```python
from build123d import *

# Parameters (mm, degrees)
ESQUISSE1_W        = 8
ESQUISSE1_H        = 8
ESQUISSE1_R        = 2.825
BOSS_EXTRU_1_DEPTH = 6


with BuildPart() as part:
    # Esquisse1 → Boss.-Extru.1 (new body)
    # profile 1 of 6: a face of its own
    with BuildSketch(Plane(origin=(0, 0, 0), x_dir=(1, 0, 0), z_dir=(0, 1, 0))):
        Rectangle(ESQUISSE1_W, ESQUISSE1_H)
        Circle(ESQUISSE1_R, mode=Mode.SUBTRACT)
    # profile 2 of 6: a face of its own
    with BuildSketch(Plane(origin=(0, 0, 0), x_dir=(1, 0, 0), z_dir=(0, 1, 0))):
        Polygon((1.6, -4), (-1.6, -4), (0, -5.7), align=None)
    # profile 3 of 6: a face of its own
    with BuildSketch(Plane(origin=(0, 0, 0), x_dir=(1, 0, 0), z_dir=(0, 1, 0))):
        Polygon((-1.6, 4), (-4, 4), (-4, 1.6), (-4, -1.6), (-4, -4), (-1.6, -4), (1.6, -4), (4, -4), (4, 4), (1.6, 4), align=None)
        with BuildLine():
            ThreePointArc((1.708252031, -2.25), (-2.825, 0), (1.708252031, 2.25))
            ThreePointArc((1.708252031, 2.25), (2.530458159, 1.255948449), (2.825, 0))
            ThreePointArc((2.825, 0), (2.530458159, -1.255948449), (1.708252031, -2.25))
        make_face(mode=Mode.SUBTRACT)
    # profile 4 of 6: a face of its own
    with BuildSketch(Plane(origin=(0, 0, 0), x_dir=(1, 0, 0), z_dir=(0, 1, 0))):
        with BuildLine():
            ThreePointArc((2.825, 0), (2.530458159, 1.255948449), (1.708252031, 2.25))
            Line((1.708252031, 2.25), (1.708252031, -2.25))
            ThreePointArc((1.708252031, -2.25), (2.530458159, -1.255948449), (2.825, 0))
        make_face()
    # profile 5 of 6: a face of its own
    with BuildSketch(Plane(origin=(0, 0, 0), x_dir=(1, 0, 0), z_dir=(0, 1, 0))):
        Polygon((-4, -1.6), (-4, 1.6), (-5.7, 0), align=None)
    # profile 6 of 6: a face of its own
    with BuildSketch(Plane(origin=(0, 0, 0), x_dir=(1, 0, 0), z_dir=(0, 1, 0))):
        Polygon((0, 5.7), (-1.6, 4), (1.6, 4), align=None)
    extrude(amount=BOSS_EXTRU_1_DEPTH)


solid = part.part
```
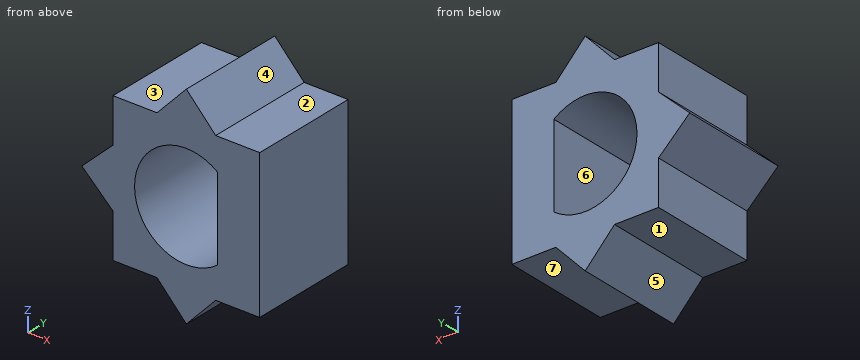
Could you check a few things on this model? Use its own coordinates, in mm. Face numbers are marked on the shaded views. A direction names the side the tool comes from. Round coordinates to 2 decimals unless told otherwise and drop trailing zeros. Loops run counter-clockwise (first coordinate to the right, second up) from the corner with the lowest first, then second, coordinate; pieces in that order, holes last. Notation, with made-up numbers: (7.25, 75.25) - (18.25, 75.25) arc R27 ccw to (18.25, 100.25) - close; hole circle Ø3 at (56.25, 68.25). An arc over 180 degrees is marked (long way). Use CSV: the item, a comma, the result in double quotes.
Item 1: If we section it at C-C on y = 1.5: List the corners of the cut face in (x, z) for me (3 decimals), then the cut area to 3 significant figures.
Here are the results:
outline,"(-5.7, 0) - (-4, -1.6) - (-4, -4) - (-1.6, -4) - (0, -5.7) - (1.6, -4) - (4, -4) - (4, 4) - (1.6, 4) - (0, 5.7) - (-1.6, 4) - (-4, 4) - (-4, 1.6) - close; hole (1.708, -2.25) - (1.708, 2.25) arc R2.825 ccw (long way) to start"
area,"50.6 mm²"
Item 2: If we section it at D-D on z = 4.75: List the corners of the cut face in (x, y) for me, then the cut area to 3 significant figures.
Here are the results:
outline,"(-0.89, 0) - (0.89, 0) - (0.89, 6) - (-0.89, 6) - close"
area,"10.7 mm²"
Item 3: If we section it at A-A on x = -0.75: List the corners of the cut face in (y, z) for me, then the cut area to 3 significant figures.
Here are the results:
outline,"(0, -4.9) - (6, -4.9) - (6, -2.72) - (0, -2.72) - close; (0, 2.72) - (6, 2.72) - (6, 4.9) - (0, 4.9) - close"
area,"26.2 mm²"
Item 4: For the marked faces 1, 2 and 3, which set-ups out of +Z, -Z, +X, -X, +Y, -Y let a thin tool reach every point of the face, with its end or its side?
Here are the results:
face 1,"-Z, -X, +Y, -Y"
face 2,"+Z, +X, +Y, -Y"
face 3,"+Z, -X, +Y, -Y"
Item 5: I need wall thicknesses on L1, parallel to Z at x = 3.5, y = 5.7; L2, parallel to Z at x = 0.25, y = 2.1; L3, parallel to Z at x = -2, y = 3. Which ranges of each line are inside material? Lowest first, please. Write a range as [from, to].
Here are the results:
L1,"z = [-4, 4]"
L2,"z = [-5.43, -2.81], [2.81, 5.43]"
L3,"z = [-4, -2], [2, 4]"
Item 6: If we section it at B-B on z = -1.25: List the corners of the cut face in (x, y) for me.
Here are the results:
outline,"(-4.37, 0) - (-2.53, 0) - (-2.53, 6) - (-4.37, 6) - close; (1.71, 0) - (4, 0) - (4, 6) - (1.71, 6) - close"
Item 7: If we mould it in two halves opening along X, with no side actions, what happens to the marked faces 4, 5, 6 and 7? For each: pulls with the +X half, pulls with the -X half, needs draft (parallel to the pull), parting line crosses it, or undercut.
Here are the results:
face 4,"pulls with the +X half"
face 5,"pulls with the -X half"
face 6,"undercut"
face 7,"needs draft"
Item 8: Will these pins go through, and if not, where does the flat tip stop? pin 1 (3 mm diameter, centred on y = 4, z = 2.5, fed in from -X); pin 2 (1 mm diameter, centred on y = 5, z = -3.5, fed in from -X); pin 3 (3.5 mm diameter, centred on y = 4.5, z = -1, fed in from -X); pin 4 (1.9 mm diameter, centred on y = 4.5, z = -2.5, fed in from -X).
Here are the results:
pin 1,"stops at x = -4.64"
pin 2,"stops at x = -4"
pin 3,"stops at x = -5.7"
pin 4,"stops at x = -4.05"
